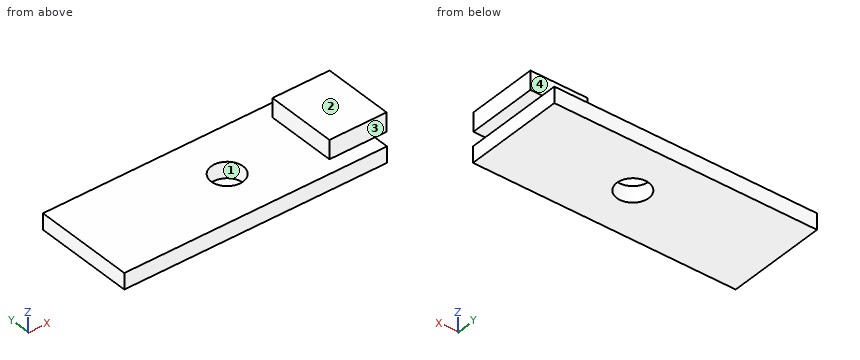
```python
from build123d import *

# Parameters (mm, degrees)
SKETCH1_W           = 28
SKETCH1_H           = 10.7
BOSS_EXTRUDE1_DEPTH = 1.7
SKETCH2_R           = 1.7
CUT_EXTRUDE1_DEPTH  = 16.083517494
SKETCH3_W           = 6.09
SKETCH3_H           = 7.5
BOSS_EXTRUDE2_DEPTH = 2


with BuildPart() as part:
    # Sketch1 → Boss-Extrude1 (new body)
    with BuildSketch(Plane.XY):
        Rectangle(SKETCH1_W, SKETCH1_H)
    extrude(amount=BOSS_EXTRUDE1_DEPTH)

    # Sketch2 → Cut-Extrude1 (cut, through all)
    with BuildSketch(Plane.XY.offset(1.7)):
        with Locations((1.3, 0)):
            Circle(SKETCH2_R)
    extrude(amount=-CUT_EXTRUDE1_DEPTH, mode=Mode.SUBTRACT)

    # Sketch3 → Boss-Extrude2 (add)
    with BuildSketch(Plane.XY.offset(1.7)):
        with Locations((12.205, 0)):
            Rectangle(SKETCH3_W, SKETCH3_H)
    extrude(amount=BOSS_EXTRUDE2_DEPTH)


solid = part.part
```
Part model, mm, in its own coordinate system. Face numbers are marked on the shaded views. Give positions to 0.01 mm unless a question says otherwise; leave off trailing zeros. Loops run counter-clockwise (first coordinate to the right, second up) from the corner with the lowest first, then second, coordinate; pieces in that order, holes last. Notation, with made-up numbers: M 40,85.5 L 86,85.5 A11 ccw 86,101.5 Z; hole C 76,-2 d2. An arc over 180 degrees is marked long. Return JSON: item names as keys, results as strings.
1) Saw through at D-D, the plane y = -2. List the corners of the cut face in (x, z).
Calculated:
{"outline": "M -14,0 L 14,0 L 14,1.7 L 15.25,1.7 L 15.25,3.7 L 9.16,3.7 L 9.16,1.7 L -14,1.7 Z"}
2) Saw through at A-A, the plane y = 0. List the corners of the cut face in (x, z), then the cut area to 3 significant figures.
Calculated:
{"outline": "M -14,0 L -0.4,0 L -0.4,1.7 L -14,1.7 Z; M 3,0 L 14,0 L 14,1.7 L 15.25,1.7 L 15.25,3.7 L 9.16,3.7 L 9.16,1.7 L 3,1.7 Z", "area": "54.0 mm2"}
3) Drill centre lines: line 1 (Y direction, x = 1.3, z = 1.25); line 2 (X direction, y = 3.25, z = 3.05); line 3 (Z direction, x = -0.5, y = 2). Where is each one in solid material? Low to high.
Calculated:
{"line 1": "y = -5.35 to -1.7, 1.7 to 5.35", "line 2": "x = 9.16 to 15.25", "line 3": "z = 0 to 1.7"}
4) Saw through at C-C, the plane z = 0.3. List the corners of the cut face in (x, y), then the cut area to 3 significant figures.
Calculated:
{"outline": "M -14,-5.35 L 14,-5.35 L 14,5.35 L -14,5.35 Z; hole C 1.3,0 d3.4", "area": "291 mm2"}
5) Saw through at B-B, the plane x = 1.3. List the corners of the cut face in (y, z), then the cut area to 3 significant figures.
Calculated:
{"outline": "M -5.35,0 L -1.7,0 L -1.7,1.7 L -5.35,1.7 Z; M 1.7,0 L 5.35,0 L 5.35,1.7 L 1.7,1.7 Z", "area": "12.4 mm2"}
6) Pull direction Y, two halves, no side cores. Call the marked faces 1, 2, 3 and 4: released by +Y, released by -Y, zero draft, split by the parting line, or undercut.
Calculated:
{"face 1": "undercut", "face 2": "zero draft", "face 3": "released by -Y", "face 4": "released by +Y"}
7) Flat gauge pins, fed straight in: pin 1 Ø2 at (x, z) = (-7.5, 3) entering from +Y; pin 2 Ø1.6 at (x, z) = (11, 3) entering from -Y; pin 3 Ø0.6 at (x, y) = (14.5, 1) entering from -Z; pin 4 Ø1 at (y, z) = (1, 3) entering from -X. Where does each tip first touch, or does it go through?
Calculated:
{"pin 1": "passes through", "pin 2": "stops at y = -3.75", "pin 3": "stops at z = 1.7", "pin 4": "stops at x = 9.16"}
